Geometry: see drawing. Coordinates: mm, zero at the bounding-box minimum. A direction names the side the tool comes from. Round coordinates to 2 decimals unless told otherwise and drop trailing zeros. Write each loop counter-clockwise with the first axis right and the second up, starting at its lowest first coordinate (ties: lowest second). Pieces come first, ordered by that corner, then holes. Notation, with made-up numbers: (47, 21.25) -> (100, 21.25) arc R27 ccw to (100, 43.25) -> close; hole circle Ø11 at (74.5, 66). An arc over 180 degrees is marked (long way). Write item = value, one per line.
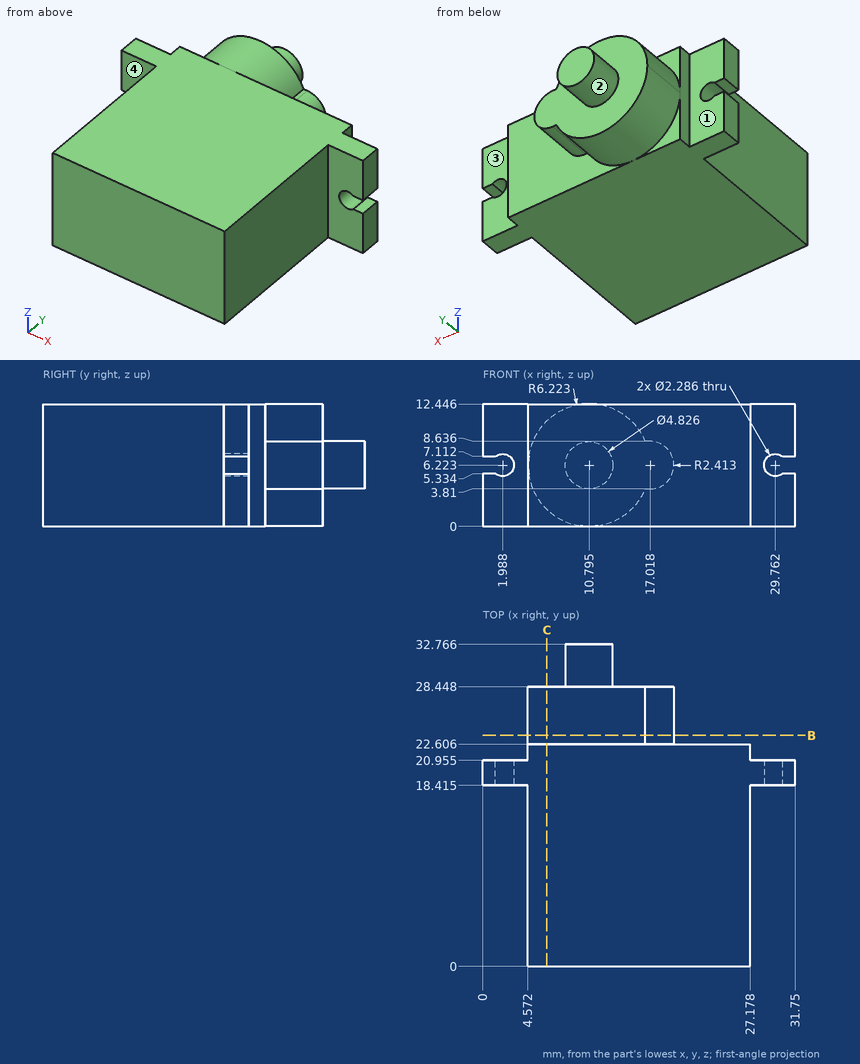
1) Cut plane C-C (x = 6.5). Return the cut outline in (y, z), and give its area (3 significant figures).
Solutions:
outline = (0, 0) -> (22.61, 0) -> (22.61, 1.72) -> (28.45, 1.72) -> (28.45, 10.73) -> (22.61, 10.73) -> (22.61, 12.45) -> (0, 12.45) -> close
area = 334 mm^2
2) Line query: L1, parallel to Y at x = 19.5, z = 1; L2, parallel to X at y = 3, z = 3.5; L3, parallel to Y at x = 2, z = 10.5 (1 decimal). Output: solid intervals per line, ascending. Write a range as from..to.
Solutions:
L1 = 0..22.61
L2 = 4.57..27.18
L3 = 18.4..21
3) Cut plane B-B (y = 23.5). Return the cut outline in (x, z) (1 decimal), and give its area (3 significant figures).
Solutions:
outline = (16.5, 3.8) -> (17, 3.8) arc R2.4 ccw to (17, 8.6) -> (16.5, 8.6) arc R6.2 ccw (long way) to start
area = 132 mm^2
4) Access query for the marked faces 1, 2, 3 and 4. Directions: +Z, -Z, +X, -X, +Y, -Y. A direction counts if a zero-diameter tool reaches every point of the face in a straight line with its end or side. Return the directions, or none.
Solutions:
face_1 = +Z, -Z, -X, +Y
face_2 = +Y
face_3 = +Z, -Z, +X, +Y
face_4 = +Z, -Z, -X, -Y
5) First-contact query: P1, Ø4, axis at y = 7, z = 1.5, coming from the +X side; P2, Ø0.5, axis at y = 21.5, z = 7.5, coming from the -X side; P3, Ø3, axis at x = 1.99, z = 6.22, coming from the +Y side (3 decimals). Flat tips, straight axial feed; report the tip coordinate or a pass-through.
Solutions:
P1 = 27.18
P2 = 4.57
P3 = 20.955
